Autodesk Inventor part; units mm, degrees
ref_plane "YZ Plane" through (0, 0, 0) normal (1, 0, 0) x (0, 1, 0)
ref_plane "XZ Plane" through (0, 0, 0) normal (0, 1, 0) x (-1, 0, 0)
ref_plane "XY Plane" through (0, 0, 0) normal (0, 0, 1) x (1, 0, 0)
sketch "Sketch1" plane through (0, 0, 0) normal (0, 1, 0) x (-1, 0, 0)
  line L0 (0, 0) -> (20, 0)
  line L1 (20, 0) -> (20, -73)
  line L2 (20, -73) -> (0, -73)
  line L3 (0, -73) -> (0, 0)
  circle A0 centre (10, -36.5) radius 6.25
  dimension "d0" = 20
  dimension "d1" = 73
  dimension "d2" = 12.5
  dimension "d3" = 10
  dimension "d4" = 36.5
extrude "Extrusion1" add sketch "Sketch1" along normal blind 5
sketch "Sketch2" plane through (0, 0, 0) normal (1, 0, 0) x (0, 0, -1)
  line L0 (10, 5) -> (63, 5)
  line L1 (63, 5) -> (63, -15)
  line L2 (63, -15) -> (10, -15)
  line L3 (10, -15) -> (10, 5)
  line L4 (0, 5) -> (73, 5)
  line L5 (0, 0) -> (0, 5)
  line L6 (73, 0) -> (73, 5)
  line L7 (73, 0) -> (0, 0)
  dimension "d7" = 10
  dimension "d8" = 10
  dimension "d9" = 15
extrude "Extrusion2" add sketch "Sketch2" along normal blind 10 contours L0 L1 L7 L3 | L7 L1 L2 L3
sketch "Sketch3" plane through (0, -15, -10) normal (0, 0, 1) x (1, 0, 0)
  line L0 (0, 10) -> (10, 10)
  line L1 (10, 10) -> (10, 0)
  line L2 (10, 0) -> (0, 0)
  line L3 (0, 0) -> (0, 10)
  line L4 (10, 20) -> (10, 0)
  line L5 (0, 0) -> (10, 0)
  point P0 (0, 15)
  dimension "d12" = 10
  dimension "d13" = 10
extrude "Extrusion3" add sketch "Sketch3" along normal blind 10
sketch "Sketch4" plane through (0, 0, 0) normal (0, -1, 0) x (1, 0, 0)
  line L0 (-20, -10) -> (0, -10)
  line L1 (0, -10) -> (0, 0)
  line L2 (0, 0) -> (-20, 0)
  line L3 (-20, 0) -> (-20, -10)
  line L4 (0, 0) -> (-20, 0)
  line L5 (-20, 0) -> (-20, -73)
  line L6 (0, -63) -> (0, 0)
  dimension "d16" = 10
extrude "Extrusion4" add sketch "Sketch4" along normal blind 15
sketch "Sketch5" plane through (0, -15, -63) normal (0, 0, -1) x (-1, 0, 0)
  line L0 (-10, 0) -> (-10, 10)
  line L1 (-10, 0) -> (-10, 10)
  line L2 (0, 10) -> (-10, 10)
  line L3 (-10, 10) -> (0, 10)
  line L4 (0, 10) -> (0, 15)
  line L5 (0, 10) -> (0, 20)
  line L6 (0, 15) -> (20, 15)
  line L7 (-10, 0) -> (20, 0)
  line L8 (20, 15) -> (20, 0)
  line L9 (20, 0) -> (-10, 0)
  dimension "d19" = 15
extrude "Extrusion5" add sketch "Sketch5" along normal blind 10
sketch "Sketch6" plane through (0, 5, 0) normal (0, 1, 0) x (1, 0, 0)
  line L0 (-5, 58.5) -> (-15, 58.5) construction
  line L1 (-5, 61) -> (-15, 61)
  line L2 (-15, 56) -> (-5, 56)
  arc A0 (-5, 56) -> (-5, 61) centre (-5, 58.5) ccw
  arc A1 (-15, 61) -> (-15, 56) centre (-15, 58.5) ccw
  line L3 (-5, 14.5) -> (-15, 14.5) construction
  line L4 (-5, 17) -> (-15, 17)
  line L5 (-15, 12) -> (-5, 12)
  arc A2 (-5, 12) -> (-5, 17) centre (-5, 14.5) ccw
  arc A3 (-15, 17) -> (-15, 12) centre (-15, 14.5) ccw
  line L6 (-20, 0) -> (0, 0)
  line L7 (0, 73) -> (-20, 73)
  line L8 (-20, 73) -> (-20, 0)
  point P0 (-10, 58.5)
  point P1 (-10, 14.5)
  dimension "d22" = 5
  dimension "d23" = 5
  dimension "d24" = 12
  dimension "d25" = 12
  dimension "d26" = 10
  dimension "d27" = 10
  dimension "d28" = 10
  dimension "d29" = 10
extrude "Extrusion6" cut sketch "Sketch6" against normal blind 10
hole "Hole1" at (5, -5, -5) direction (0, -1, 0) diameter 4.2 end through all
hole "Hole3" at (5, -5, -68) direction (0, -1, 0) diameter 4.2 end through all
properties part number "powerSwitchHolder"
Input: part model. Units: mm. Frame: model coordinates. A direction names the side the tool comes from. Coordinates: 2 decimals unless noted, no trailing zeros. Loops run counter-clockwise (first coordinate to the right, second up) from the corner with the lowest first, then second, coordinate; pieces in that order, holes last.
Q1. Contact query for flat-ended pins moving along their axis: pin 1 (7.5 mm diameter, centred on y = -4.5, z = -48, fed in from -X); pin 2 (3 mm diameter, centred on x = -9, z = -51.5, fed in from -Y); pin 3 (5.5 mm diameter, centred on x = 5, z = -68, fed in from +Y). Output: stop coordinate, or through.
Results are:
pin 1: stops at x = 0
pin 2: stops at y = 0
pin 3: stops at y = -5
Q2. Section B-B, the plane z = -14.5. Return the cut outline in (x, y).
Results are:
outline: (-20, 0) - (-17.5, 0) - (-17.5, 5) - (-20, 5) - close; (-2.5, 0) - (0, 0) - (0, -15) - (10, -15) - (10, 5) - (-2.5, 5) - close
Q3. Mould query, pull axis Z, two halves, no side actions, for faces 6 (the flat face through (-8, -5, 0)), 7 (the flat face through (0, 0, -5)), 8 (the flat face through (0, -8, -37)). Classes: +Z half, -Z half, draft (parallel to the pull), parting line (faces both ways), or undercut.
Results are:
face 6: +Z half
face 7: draft
face 8: undercut
Q4. Line query: line 1 along Z through (x, y) = (5, -6.75); line 2 along X through (y, z) = (-11.75, -5); line 3 along Z through (x, y) = (-2.25, -1.5). Output: solid intervals per line, ascending.
Results are:
line 1: z = -73 to -70.1, -65.9 to -7.1, -2.9 to 0
line 2: x = -20 to 2.9, 7.1 to 10
line 3: z = -73 to -63, -10 to 0
Q5. Section C-C, the plane x = -10. Return the cut outline in (y, z).
Results are:
outline: (-15, -73) - (5, -73) - (5, -61) - (0, -61) - (0, -63) - (-15, -63) - close; (-15, -10) - (0, -10) - (0, -12) - (5, -12) - (5, 0) - (-15, 0) - close; (0, -56) - (5, -56) - (5, -42.75) - (0, -42.75) - close; (0, -30.25) - (5, -30.25) - (5, -17) - (0, -17) - close
Q6. Set-up query: faces 1 (the flat face through (-8, -5, -73)), 2 (the cylindrical face through (-2.5, 2.5, -14.4)), 3 (the flat face through (-10, -7, -10)), 4 (the flat face through (4.9, -5, -7.3)), 5 (the flat face through (5, 0, -63)). Return all of +Z, -Z, +X, -X, +Y, -Y with unobstructed straight access to the full face (end or side cutting, diameter ignored); none if empty.
Results are:
face 1: -Z, +X, -X, +Y, -Y
face 2: +Y, -Y
face 3: -X, -Y
face 4: +Z, +X, +Y
face 5: -Z, +X, +Y
Q7. Section A-A, the plane y = 2.5. Return the cut outline in (x, z).
Results are:
outline: (-20, -73) - (0, -73) - (0, -63) - (10, -63) - (10, -10) - (0, -10) - (0, 0) - (-20, 0) - close; hole circle Ø12.5 at (-10, -36.5); hole (-15, -61) - (-5, -61) arc R2.5 ccw to (-5, -56) - (-15, -56) arc R2.5 ccw to start; hole (-15, -17) - (-5, -17) arc R2.5 ccw to (-5, -12) - (-15, -12) arc R2.5 ccw to start
